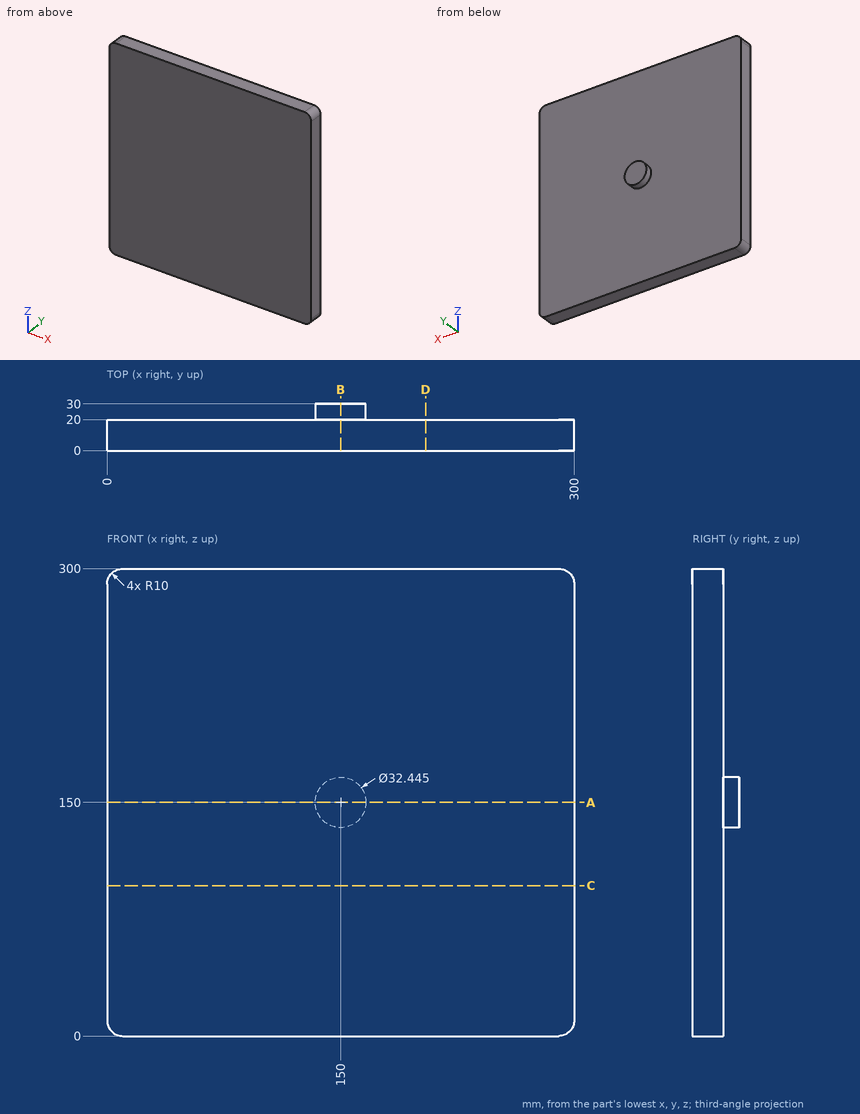
Here's the drawing with two shaded views (mm, measured from the low corner). I have some questions. Round coordinates to 2 decimals unless told otherwise and drop trailing zeros. Write each loop counter-clockwise with the first axis right and the second up, starting at its lowest first coordinate (ties: lowest second). Pieces come first, ordered by that corner, then holes. Notation, with made-up numbers: M 53,-6 L 78,-6 A34 cw 78,24 Z; hole C 1.5,68 d6. An arc over 180 degrees is marked long. Answer in a Markdown table with one row per item. Add a question column.
Q1. Imagine slicing it at D-D (x = 204.5). Please give me the cut outline in (y, z), then the cut area to 3 significant figures.
Q2. Imagine slicing it at C-C (z = 96.5). Please give me the cut outline in (x, y), then the cut area to 3 significant figures.
Q3. Imagine slicing it at A-A (z = 150). Please give me the cut outline in (x, y).
Q4. If I drill on line 1 (Y direction, x = 221.5, z = 224); line 2 (X direction, y = 26.25, z = 163); line 3 (X direction, y = 26.25, z = 158), over which ranges is the centre line in solid material (lowest first)? Write a range as from..to.
Q5. Imagine slicing it at B-B (x = 150). Please give me the cut outline in (y, z), then the cut area to 3 significant figures.
Q6. Will these pins go through, and if not, where does the flat tip stop? pin 1 Ø2 at (x, z) = (154, 149) entering from -Y; pin 2 Ø3 at (y, z) = (22, 72) entering from -X; pin 3 Ø1.5 at (x, z) = (89, 71) entering from +Y.
Values:
| question | item | result |
|---|---|---|
| 1 | outline | M 0,0 L 20,0 L 20,300 L 0,300 Z |
| 1 | area | 6,000 mm^2 |
| 2 | outline | M 0,0 L 300,0 L 300,20 L 0,20 Z |
| 2 | area | 6,000 mm^2 |
| 3 | outline | M 0,0 L 300,0 L 300,20 L 166.22,20 L 166.22,30 L 133.78,30 L 133.78,20 L 0,20 Z |
| 4 | line 1 | 0..20 |
| 4 | line 2 | 140.3..159.7 |
| 4 | line 3 | 135.89..164.11 |
| 5 | outline | M 0,0 L 20,0 L 20,133.78 L 30,133.78 L 30,166.22 L 20,166.22 L 20,300 L 0,300 Z |
| 5 | area | 6,320 mm^2 |
| 6 | pin 1 | y = 0 |
| 6 | pin 2 | through |
| 6 | pin 3 | y = 20 |
